Can you work these out from the model? Positions are in its coordinate system, mm. A direction names the side the tool comes from. Coordinates: 2 decimals unless noted, no trailing zeros. Order: outer loops, then holes, each group sorted by start corner. A loop starts at its lowest first (then second) coordinate and runs counter-clockwise, first axis right, second up. Notation, with made-up numbers: (56.5, 51) - (114.5, 51) arc R9 cw to (114.5, 60) - close; hole circle Ø1 at (-10.5, 14.25). An arc over 180 degrees is marked (long way). Return JSON: item names as keys, results as strings. Group by question number.
1) For pin 1 Ø12 at (x, y) = (4, -7.5) entering from -Z; pin 2 Ø10 at (x, z) = (-1, 17.5) entering from -Y; pin 3 Ø6 at (x, z) = (-20, -7.5) entering from -Y; pin 4 Ø10 at (y, z) = (-7, -6.5) entering from -X, each with a flat end and sliding along its axis, tell me the tip position at first contact or that it passes through.
2) If we mould it in two halves opening along Z, with no side actions, what happens to faces 1 (the face through (-0.1, -24.2, -30)), 2 (the face through (-0.704, -31.992, 20.437)), 3 (the face through (-0.1, -24.2, 16)), 4 (the face through (0, -19, -39))? For each: pulls with the +Z half, pulls with the -Z half, needs draft (parallel to the pull), parting line crosses it, or undercut.
3) Imagine slicing it at B-B (x = 28.5). Write out the boundary of the cut face in (y, z).
4) If I drill on line 1 along Z through (x, y) = (20, -11); line 2 along Z through (x, y) = (-19, -24); line 3 along X through (y, z) = (-10, -18), over which ranges is the centre line in solid material (lowest first)?
5) Imagine slicing it at C-C (z = 18.5). Write out the boundary of the cut face in (x, y), and give its area (3 significant figures).
6) Which directions (+Z, -Z, +X, -X, +Y, -Y) give clear straight access to the entire face, cutting with the end or side of a thin tool? Please do faces 5 (the face through (20, 0, -7)), 6 (the face through (-4, -22, 7)).
7) Imagine slicing it at A-A (y = -26.5). Write out the boundary of the cut face in (x, z).
8) Imagine slicing it at D-D (x = 0). Write out the boundary of the cut face in (y, z), and give its area (3 significant figures).
```python
from build123d import *

# Parameters (mm, degrees)
SKETCH1_R           = 22
SKETCH1_R_2         = 16
BOSS_EXTRUDE2_DEPTH = 7
SKETCH3_R           = 24
BOSS_EXTRUDE6_DEPTH = 9
SKETCH6_R           = 32
BOSS_EXTRUDE7_DEPTH = 9
SKETCH7_R           = 16
CUT_EXTRUDE2_DEPTH  = 56.425625842
CUT_EXTRUDE3_DEPTH  = 79.383671769


with BuildPart() as part:
    # Sketch1 → Boss-Extrude2 (new, symmetric)
    with BuildSketch(Plane.XY):
        Circle(SKETCH1_R)
        Circle(SKETCH1_R_2, mode=Mode.SUBTRACT)
    extrude(amount=BOSS_EXTRUDE2_DEPTH, both=True)

    # Sketch3 → Boss-Extrude6 (add)
    with BuildSketch(Plane.XY.offset(7)):
        Circle(SKETCH3_R)
    extrude(amount=BOSS_EXTRUDE6_DEPTH)

    # Sketch6 → Boss-Extrude7 (add)
    with BuildSketch(Plane.XY.offset(16)):
        Circle(SKETCH6_R)
    extrude(amount=BOSS_EXTRUDE7_DEPTH)

    # Sketch7 → Cut-Extrude2 (cut, through all)
    with BuildSketch(Plane(origin=(0, 0, -7), x_dir=(-1, 0, 0), z_dir=(0, 0, -1))):
        Circle(SKETCH7_R)
    extrude(amount=-CUT_EXTRUDE2_DEPTH, mode=Mode.SUBTRACT)

    # Mirror3: part across plane


with BuildPart() as part_1:
    add(part.part)
    add(part.part.mirror(Plane.XY.offset(-7)))

    # Sketch8 → Cut-Extrude3 (cut, through all)
    with BuildSketch(Plane.XY.offset(25)):
        Polygon((-194.543052514, 0), (-35.372068519, 0), (34.570182834, 0), (193.741166829, 0), (193.741166829, 318.34196799), (-194.543052514, 318.34196799), align=None)
    extrude(amount=-CUT_EXTRUDE3_DEPTH, mode=Mode.SUBTRACT)


solid = part_1.part
```
Calculated:
{
 "1": {"pin 1": "through", "pin 2": "y = -32", "pin 3": "y = -13.96", "pin 4": "x = -21.91"},
 "2": {"face 1": "undercut", "face 2": "needs draft", "face 3": "undercut", "face 4": "pulls with the -Z half"},
 "3": {"outline": "(-14.55, -39) - (0, -39) - (0, -30) - (-14.55, -30) - close; (-14.55, 16) - (0, 16) - (0, 25) - (-14.55, 25) - close"},
 "4": {"line 1": "-39 to -21, 7 to 25", "line 2": "-39 to -30, 16 to 25", "line 3": "-19.6 to -12.49, 12.49 to 19.6"},
 "5": {"outline": "(-32, 0) arc R32 ccw to (32, 0) - (16, 0) arc R16 cw to (-16, 0) - close", "area": "1,210 mm2"},
 "6": {"face 5": "+Z, -Z, +X, -X, +Y", "face 6": "-Y"},
 "7": {"outline": "(-17.94, -39) - (17.94, -39) - (17.94, -30) - (-17.94, -30) - close; (-17.94, 16) - (17.94, 16) - (17.94, 25) - (-17.94, 25) - close"},
 "8": {"outline": "(-32, -39) - (-16, -39) - (-16, 25) - (-32, 25) - (-32, 16) - (-24, 16) - (-24, 7) - (-22, 7) - (-22, -21) - (-24, -21) - (-24, -30) - (-32, -30) - close", "area": "600 mm2"}
}
